Source: CAD feature listing. Evaluate the final solid. Frame: model axes, mm. Face numbers are marked on the shaded views. A direction names the side the tool comes from. Round coordinates to 2 decimals unless told otherwise and drop trailing zeros. Loops run counter-clockwise (first coordinate to the right, second up) from the corner with the lowest first, then second, coordinate; pieces in that order, holes last. Notation, with made-up numbers: M -6.5,86.5 L 40.5,86.5 A21 cw 40.5,117.5 Z; hole C 52.25,82.25 d1. An arc over 180 degrees is marked long. One line per item, written item: value.
Autodesk Inventor part; units mm, degrees
ref_plane "YZ Plane" through (0, 0, 0) normal (1, 0, 0) x (0, 1, 0)
ref_plane "XZ Plane" through (0, 0, 0) normal (0, 1, 0) x (-1, 0, 0)
ref_plane "XY Plane" through (0, 0, 0) normal (0, 0, 1) x (1, 0, 0)
sketch "Esquisse1" plane through (0, 0, 0) normal (0, 1, 0) x (-1, 0, 0)
  line L0 (-20, 30) -> (20, 30)
  line L1 (20, 30) -> (20, -30)
  line L2 (20, -30) -> (-20, -30)
  line L3 (-20, -30) -> (-20, 30)
  line L4 (-20, 30) -> (20, -30) construction
  line L5 (20, 30) -> (-20, -30) construction
  point P0 (0, 0)
  dimension "d0" = 40
  dimension "d1" = 60
extrude "Extrusion1" add sketch "Esquisse1" along normal mid plane 56.5
sketch "Esquisse2" plane through (20, 28.25, -30) normal (0, 0, -1) x (-1, 0, 0)
  line L0 (0, 0) -> (40, 0)
  line L1 (16, 0) -> (16, -7)
  line L2 (16, -7) -> (12, -7)
  line L3 (12, -7) -> (12, -15)
  line L4 (20, 0.6313) -> (20, -19.069)
  line L5 (12, -15) -> (20, -15)
  line L6 (24, 0) -> (24, -7)
  line L7 (24, -7) -> (28, -7)
  line L8 (28, -7) -> (28, -15)
  line L9 (28, -15) -> (20, -15)
  point P0 (20, -28.25)
  point P1 (20, 0)
  dimension "d4" = 7
  dimension "d5" = 4
  dimension "d6" = 4
  dimension "d7" = 8
extrude "Extrusion2" cut sketch "Esquisse2" against normal through all
sketch "Esquisse3" plane through (-20, -28.25, 30) normal (0, 0, 1) x (1, 0, 0)
  line L0 (40, 0) -> (40, 56.5)
  line L1 (0, 25) -> (40, 25)
  line L2 (40, 25) -> (40, 0)
  line L3 (40, 0) -> (0, 0)
  line L4 (0, 0) -> (0, 25)
  line L5 (0, 25) -> (40, 0) construction
  line L6 (40, 25) -> (0, 0) construction
  point P0 (20, 28.25)
  point P1 (20, 12.5)
  dimension "d10" = 25
extrude "Extrusion3" add sketch "Esquisse3" along normal blind 30
fillet "Congé1" radius 2 6 edges at (20, -3.25, 45) (20, -15.75, 60) (0, -3.25, 60) (-20, -3.25, 45) (-20, -15.75, 60) (0, -28.25, 60)
sketch "Esquisse4" plane through (-18, -3.25, 30) normal (0, 1, 0) x (1, 0, 0)
  line L0 (0, -28) -> (0, 0)
  line L1 (36, -28) -> (0, -28)
  line L2 (36, 0) -> (36, -28)
  line L3 (0, 0) -> (36, 0)
  line L4 (46, 30) -> (-10, 30)
  point P0 (18, 30)
  point P1 (18.2732, -15)
  dimension "d21" = 45
hole "Perçage1" at (0.2732, -3.25, 45) direction (0, -1, 0) diameter 16 end through all
mirror "Mise en miroir2" about plane through (0, 0, 0) normal (0, 0, 1) of "Extrusion3", "Congé1", "Perçage1"
properties part number "SupportFrein"
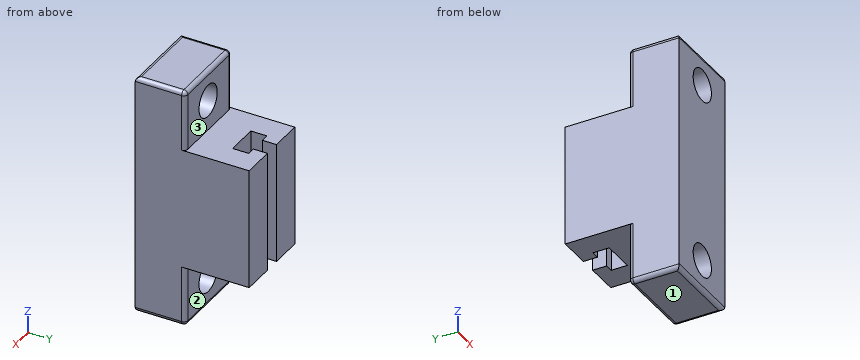
1. Ray query, line 1 (Y direction, x = 7, z = -8.5); line 2 (Z direction, x = 5, y = -21); line 3 (X direction, y = -13.25, z = -45). Return the intervals inside material, ascending. Write a range as [from, to].
Report:
line 1: y = [-28.25, 13.25], [21.25, 28.25]
line 2: z = [-60, -51.45], [-38.55, 38.55], [51.45, 60]
line 3: x = [-20, -7.73], [8.27, 20]
2. Section query D-D (z = -14). Return the cut outline in (x, y), and give its area (3 significant figures).
Report:
outline: M -20,-28.25 L 20,-28.25 L 20,28.25 L 4,28.25 L 4,21.25 L 8,21.25 L 8,13.25 L -8,13.25 L -8,21.25 L -4,21.25 L -4,28.25 L -20,28.25 Z
area: 2,080 mm2
3. Section query C-C (x = -2). Return the cut outline in (y, z).
Report:
outline: M -28.25,-58 A2 ccw -26.25,-60 L -5.25,-60 A2 ccw -3.25,-58 L -3.25,-52.67 L -28.25,-52.67 Z; M -28.25,-37.33 L -3.25,-37.33 L -3.25,-30 L 13.25,-30 L 13.25,30 L -3.25,30 L -3.25,37.33 L -28.25,37.33 Z; M -28.25,52.67 L -3.25,52.67 L -3.25,58 A2 ccw -5.25,60 L -26.25,60 A2 ccw -28.25,58 Z
4. Reachability of the marked faces 1, 2 and 3 from +Z, -Z, +X, -X, +Y, -Y: full face, straight path, thin tool, end or side. Return the list, or none.
Report:
face 1: -Z, +X, -X, +Y, -Y
face 2: -Z, +X, -X, +Y
face 3: +Z, +X, -X, +Y
5. Section query A-A (y = 22.5). Return the cut outline in (x, z).
Report:
outline: M -20,-30 L -4,-30 L -4,30 L -20,30 Z; M 4,-30 L 20,-30 L 20,30 L 4,30 Z
6. Pin query (flat end, axial travel): pin 1 (1 mm diameter, centred on x = -14.5, y = 11.5, fed in from -Z); pin 2 (14 mm diameter, centred on x = 3, z = -45.5, fed in from +Y); pin 3 (10 mm diameter, centred on x = -7, y = 15.5, fed in from +Z). Return the tip coordinate at first contact, or that it passes through.
Report:
pin 1: stops at z = -30
pin 2: stops at y = -3.25
pin 3: stops at z = 30
7. Section query B-B (z = 45). Return the cut outline in (x, y).
Report:
outline: M -20,-28.25 L -7.73,-28.25 L -7.73,-3.25 L -18,-3.25 A2 ccw -20,-5.25 Z; M 8.27,-28.25 L 20,-28.25 L 20,-5.25 A2 ccw 18,-3.25 L 8.27,-3.25 Z
